For this review, take the finished solid that the model builds, in its own axes (mm). A direction names the side the tool comes from. Give positions to 0.01 mm unless a question says otherwise; leave off trailing zeros. Write each loop counter-clockwise with the first axis right and the second up, starting at its lowest first coordinate (ties: lowest second). Pieces come first, ordered by that corner, then holes.
1) Machinability: for faces 4 (the face through (0, 27, 0)), 5 (the face through (-11, 6, -6)), which of the approach directions +Z, -Z, +X, -X, +Y, -Y give a long, thin tool a straight path to every point of the face, cutting with its end or side? Answer none if there is none.
2) We need section A-A on x = 0. Give the boundary of the cut face in (y, z).
3) Wall thickness on line 1 along X through (y, z) = (3.15, -6.5); line 2 along Z through (x, y) = (12, 2.25); line 3 along Z through (x, y) = (0.5, 25.5): over which ranges is each line inside the solid? List them lowest first.
4) For P1, Ø1, axis at x = 5.5, y = 18.5, coming from the -Z side; P2, Ø8, axis at y = 18.5, z = -7.5, coming from the +X side; P3, Ø4, axis at y = 20, z = 2.5, coming from the +X side, all flat-tipped, find the tip position at first contact; note any pin that passes through.
5) We need section C-C on y = 24. Give the boundary of the cut face in (x, z).
6) We need section B-B on z = 13. Give the boundary of the cut face in (x, y), and give its area (3 significant figures).
7) We need section D-D on y = 2.5. Give the boundary of the cut face in (x, z).
8) Draft analysis for pull direction X (two halves, no side actions). For faces 1 (the face through (0, 0, 0)), 2 (the face through (-19.524, 13.311, -4.336)), 3 (the face through (0.07, 2.96, 14.5)), state which applies: pulls with the +X half, pulls with the -X half, needs draft (parallel to the pull), parting line crosses it, or undercut.
from build123d import *

# Parameters (mm, degrees)
SKETCH1_R           = 20
BOSS_EXTRUDE1_DEPTH = 27
SKETCH2_R           = 1.5
CUT_EXTRUDE1_DEPTH  = 6


with BuildPart() as part:
    # Sketch1 → Boss-Extrude1 (new body)
    with BuildSketch(Plane(origin=(0, 0, 0), x_dir=(1, 0, 0), z_dir=(0, 1, 0))):
        with Locations(Location((0, 0, 0), (0, 0, 270))):
            Circle(SKETCH1_R)
    extrude(amount=BOSS_EXTRUDE1_DEPTH)

    # Sketch2 → Cut-Extrude1 (cut)
    with BuildSketch(Plane.XZ):
        with Locations(Location((0, 13, 0), (0, 0, 270))):
            Circle(SKETCH2_R)
        with Locations(Location((11.258330249, -6.5, 0), (0, 0, 270))):
            Circle(SKETCH2_R)
        with Locations(Location((-11.258330249, -6.5, 0), (0, 0, 270))):
            Circle(SKETCH2_R)
    extrude(amount=-CUT_EXTRUDE1_DEPTH, mode=Mode.SUBTRACT)


solid = part.part
Results list:
1. face 4: +Z, -Z, +X, -X, +Y
1. face 5: -Y
2. outline: (0, -20) - (27, -20) - (27, 20) - (0, 20) - (0, 14.5) - (6, 14.5) - (6, 11.5) - (0, 11.5) - close
3. line 1: x = -18.91 to -12.76, -9.76 to 9.76, 12.76 to 18.91
3. line 2: z = -16 to -7.8, -5.2 to 16
3. line 3: z = -19.99 to 19.99
4. P1: stops at z = -19.36
4. P2: stops at x = 19.69
4. P3: stops at x = 19.99
5. outline: circle Ø40 at (0, 0)
6. outline: (-15.2, 0) - (-1.5, 0) - (-1.5, 6) - (1.5, 6) - (1.5, 0) - (15.2, 0) - (15.2, 27) - (-15.2, 27) - close
6. area: 803 mm2
7. outline: circle Ø40 at (0, 0); hole circle Ø3 at (-11.26, -6.5); hole circle Ø3 at (0, 13); hole circle Ø3 at (11.26, -6.5)
8. face 1: needs draft
8. face 2: parting line crosses it
8. face 3: undercut
